from build123d import *

# Parameters (mm, degrees)
EXTRUDE1_DEPTH = 5


with BuildPart() as part:
    # Sketch1 → Extrude1 (new body)
    with BuildSketch(Plane.XY):
        with BuildLine():
            Line((9.001968821, -4.537365816), (93.001968821, -46.87685134))
            ThreePointArc((93.001968821, -46.87685134), (98.008613867, -50.462021725), (101.687244374, -55.40040394))
            ThreePointArc((101.687244374, -55.40040394), (102.79133326, -56.569164438), (104.34033103, -57))
            Line((104.34033103, -57), (123.176722972, -57))
            ThreePointArc((123.176722972, -57), (124.918831839, -56.442346555), (126.013278698, -54.976704463))
            Line((126.013278698, -54.976704463), (140.410371512, -13.164510908))
            ThreePointArc((140.410371512, -13.164510908), (141.225712031, -9.954099936), (141.5, -6.653147818))
            Line((141.5, -6.653147818), (141.5, 12))
            ThreePointArc((141.5, 12), (140.621320344, 14.121320344), (138.5, 15))
            Line((138.5, 15), (128.260336739, 15))
            ThreePointArc((128.260336739, 15), (127.204940422, 14.808226952), (126.284475151, 14.257425743))
            ThreePointArc((126.284475151, 14.257425743), (101.948595314, 3.0109904), (75.399274569, 6.732673267))
            ThreePointArc((75.399274569, 6.732673267), (74.794571806, 6.932406844), (74.161334016, 7))
            Line((74.161334016, 7), (44.749434711, 7))
            ThreePointArc((44.749434711, 7), (42.436200432, 7.271230953), (40.2484503, 8.070210566))
            Line((40.2484503, 8.070210566), (28.623258855, 13.929789434))
            ThreePointArc((28.623258855, 13.929789434), (26.435508723, 14.728769047), (24.122274444, 15))
            Line((24.122274444, 15), (-28.250565289, 15))
            ThreePointArc((-28.250565289, 15), (-30.563799568, 14.728769047), (-32.7515497, 13.929789434))
            Line((-32.7515497, 13.929789434), (-44.376741145, 8.070210566))
            ThreePointArc((-44.376741145, 8.070210566), (-46.564491277, 7.271230953), (-48.877725556, 7))
            Line((-48.877725556, 7), (-66.5, 7))
            ThreePointArc((-66.5, 7), (-70.035533906, 5.535533906), (-71.5, 2))
            Line((-71.5, 2), (-71.5, -6.015697791))
            ThreePointArc((-71.5, -6.015697791), (-72.210213011, -9.717029673), (-74.23997154, -12.892614743))
            Line((-74.23997154, -12.892614743), (-86.801586013, -26.154033952))
            ThreePointArc((-86.801586013, -26.154033952), (-87.591784672, -27.781510557), (-87.302514305, -29.56740436))
            Line((-87.302514305, -29.56740436), (-82.850295323, -38.400444957))
            ThreePointArc((-82.850295323, -38.400444957), (-81.110849912, -39.899247013), (-78.82106317, -39.729086464))
            Line((-78.82106317, -39.729086464), (-9.001968821, -4.537365816))
            ThreePointArc((-9.001968821, -4.537365816), (0, -2.396944684), (9.001968821, -4.537365816))
        make_face()
    extrude(amount=EXTRUDE1_DEPTH)


solid = part.part
Part model, mm, in its own coordinate system. A direction names the side the tool comes from. Give positions to 0.01 mm unless a question says otherwise; leave off trailing zeros. Loops run counter-clockwise (first coordinate to the right, second up) from the corner with the lowest first, then second, coordinate; pieces in that order, holes last. Notation, with made-up numbers: (25.25, 45.25) -> (59.25, 45.25) arc R19 cw to (59.25, 70.25) -> close; hole circle Ø1 at (6.5, 2.5). An arc over 180 degrees is marked (long way). Write each question's results on one line, items separated by ' | '. Start each with the question number.
Q1. Band-saw the part on C-C on y = -42. List the corners of the cut face in (x, z), plus the area to 3 significant figures.
Q2. Wall check: L1, parallel to Y at x = 9, z = 2.3; L2, parallel to X at y = -7.5, z = 3.3; L3, parallel to X at y = -10.5, z = 3.55. Give the ranges that are in metal, low to high.
Q3. Pull direction X, two halves, no side cores. Call faces 1 (the face through (97.947, -50.402, 2.465)), 2 (the face through (34.517, 10.959, 2.465)), 3 (the face through (133, 15, 2)): +X half, -X half, draft (parallel to the pull), parting line (faces both ways), or undercut.
Q4. Which spindle directions (+Z, -Z, +X, -X, +Y, -Y) get a long thin tool onto all of the face, cutting with end or side? Do faces 4 (the face through (-44.4, -22.38, 2.46)), 5 (the face through (26.47, 14.72, 2.46)), 6 (the face through (-58, 7, 2)), 7 (the face through (141.22, -10, 2.46)). Say none if no direction does.
Q5. Pin check, flat tips, straight feed: P1, Ø2.5, axis at x = -54.5, z = 2, coming from the +Y side; P2, Ø1.5, axis at x = 14.5, z = 1.5, coming from the -Y side; P3, Ø3, axis at y = -38.5, z = 2.5, coming from the +X side. Stop position of each tip, or through.
Q6. Band-saw the part on B-B on x = 65.5. List the corners of the cut face in (y, z).
Results are:
1) outline: (83.33, 0) -> (130.48, 0) -> (130.48, 5) -> (83.33, 5) -> close | area: 236 mm²
2) L1: y = -4.54 to 15 | L2: x = -71.61 to -14.88, 14.88 to 141.48 | L3: x = -72.56 to -20.83, 20.83 to 141.13
3) face 1: -X half | face 2: undercut | face 3: draft
4) face 4: +Z, -Z, -Y | face 5: +Z, -Z, +Y | face 6: +Z, -Z, -X, +Y | face 7: +Z, -Z, +X, -Y
5) P1: stops at y = 7 | P2: stops at y = -7.69 | P3: stops at x = 132.2
6) outline: (-33.01, 0) -> (7, 0) -> (7, 5) -> (-33.01, 5) -> close
